Geometry check sheet. Reference: the model listing, model coordinates, mm. A direction names the side the tool comes from. Give positions to 0.01 mm unless a question says otherwise; leave off trailing zeros. Order: outer loops, then holes, each group sorted by start corner. A loop starts at its lowest first (then second) coordinate and runs counter-clockwise, first axis right, second up.
from build123d import *

# Parameters (mm, degrees)
F0_R     = 20
F0_R_2   = 14.5
F1_DEPTH = 3
F0_R_3   = 12.5
F2_DEPTH = 20
F3_R     = 13.014075
F4_DEPTH = 4
F5_R     = 6


with BuildPart() as f1:
    # F0 (on Top) → F1 (new body)
    with BuildSketch(Plane.XY):
        Circle(F0_R)
        Circle(F0_R_2, mode=Mode.SUBTRACT)
    extrude(amount=F1_DEPTH)

    # F0 (on Top) → F2 (join)
    with BuildSketch(Plane.XY):
        Circle(F0_R_2)
        Circle(F0_R_3, mode=Mode.SUBTRACT)
    extrude(amount=F2_DEPTH)

    # F3 (on face) → F4 (join)
    with BuildSketch(Plane.XY.offset(20)):
        Circle(F3_R)
    extrude(amount=-F4_DEPTH)

    # F5
    f5_edges = [f1.edges().sort_by_distance(p)[0] for p in [
        (-14.5, 0, 20),
    ]]
    fillet(f5_edges, radius=F5_R)


solid = f1.part
Item 1: Gauge pin test, flat ends, axial feed: pin 1 (4 mm diameter, centred on x = 14.5, z = 7.5, fed in from -Y); pin 2 (8 mm diameter, centred on x = -14, y = 4, fed in from +Z); pin 3 (8 mm diameter, centred on x = -4, z = 9.5, fed in from -Y). Record the tip position at first contact, or that the pin passes through.
Reported:
pin 1: stops at y = -7.35
pin 2: stops at z = 19.64
pin 3: stops at y = -14.5
Item 2: Draft check along Y on faces 4 (the cylindrical face through (6.691, -12.864, 8.423)), 5 (the flat face through (9, 9, 0)), 6 (the cylindrical face through (11.923, 3.755, 7.888)). Enter one of: released by +Y, released by -Y, zero draft, split by the parting line, or undercut.
Reported:
face 4: split by the parting line
face 5: zero draft
face 6: undercut
Item 3: Sectioned sample at C-C (z = 12). Enter the section's corners in (x, y), and give its area (3 significant figures).
Reported:
outline: circle Ø29 at (0, 0); hole circle Ø25 at (0, 0)
area: 170 mm2
Item 4: Sectioned sample at A-A (y = 0). Enter the section's corners in (x, z).
Reported:
outline: (-20, 0) - (-12.5, 0) - (-12.5, 16) - (12.5, 16) - (12.5, 0) - (20, 0) - (20, 3) - (14.5, 3) - (14.5, 14) arc R6 ccw to (8.5, 20) - (-8.5, 20) arc R6 ccw to (-14.5, 14) - (-14.5, 3) - (-20, 3) - close
Item 5: Sectioned sample at D-D (z = 15.25). Enter the section's corners in (x, y), and give its area (3 significant figures).
Reported:
outline: circle Ø28.74 at (0, 0); hole circle Ø25 at (0, 0)
area: 158 mm2
Item 6: Set-up check for faces 1 (the cylindrical face through (-4.336, -19.524, 1.479)), 2 (the flat face through (10.3, 10.5, 3)), 3 (the flat face through (0, 0, 16)): record each of +Z, -Z, +X, -X, +Y, -Y from which the full face is reachable in a straight line by a thin tool's end or side.
Reported:
face 1: +Z, -Z
face 2: +Z
face 3: -Z
Item 7: Scan lines: L1, parallel to Y at x = 0, z = 11; L2, parallel to Z at x = -0.5, y = -5; L3, parallel to Z at x = 2.5, y = 15.5. Record each from-to range of solid material in increasing order.
Reported:
L1: y = -14.5 to -12.5, 12.5 to 14.5
L2: z = 16 to 20
L3: z = 0 to 3
